```python
from build123d import *

# Parameters (mm, degrees)
ESTRUSIONE_ESTRUSIONE1_DEPTH    = 5
SCHIZZO5_R                      = 1.75
SCHIZZO5_R_2                    = 10
SCHIZZO5_R_3                    = 11
SCHIZZO5_R_4                    = 13
SCHIZZO5_R_5                    = 26
SCHIZZO5_W                      = 37
SCHIZZO5_H                      = 24
TAGLIO_ESTRUSIONE2_DEPTH        = 7
SCHIZZO6_R                      = 4
TAGLIO_ESTRUSIONE3_DEPTH        = 10
FORI_ALESATO_4_0MM1_D           = 4
FORI_ALESATO_4_0MM1_DEPTH       = 40.6
FORI_ALESATO_4_0MM1_CSINK_D     = 4.05
FORI_ALESATO_4_0MM1_CSINK_ANGLE = 90
FORI_ALESATO_4_0MM1_TIP         = 1.201721238


with BuildPart() as part:
    # Schizzo1 → Estrusione-Estrusione1 (new body)
    with BuildSketch(Plane.XY):
        with BuildLine():
            Line((0, 8), (0, 185))
            ThreePointArc((0, 185), (2.343145751, 190.656854249), (8, 193))
            Line((8, 193), (179, 193))
            ThreePointArc((179, 193), (184.656854249, 190.656854249), (187, 185))
            Line((187, 185), (187, 149.313708499))
            ThreePointArc((187, 149.313708499), (186.39103626, 146.25224104), (184.656854249, 143.656854249))
            Line((184.656854249, 143.656854249), (43.343145751, 2.343145751))
            ThreePointArc((43.343145751, 2.343145751), (40.74775896, 0.60896374), (37.686291501, 0))
            Line((37.686291501, 0), (8, 0))
            ThreePointArc((8, 0), (2.343145751, 2.343145751), (0, 8))
        make_face()
    extrude(amount=ESTRUSIONE_ESTRUSIONE1_DEPTH)

    # Schizzo5 → Taglio-Estrusione2 (cut)
    with BuildSketch(Plane.XY.offset(5)):
        with Locations((10, 90)):
            Circle(SCHIZZO5_R)
        with Locations((54.5, 90)):
            Circle(SCHIZZO5_R)
        with Locations((83.5, 161)):
            Circle(SCHIZZO5_R_2)
        with Locations((106.319509986, 90)):
            Circle(SCHIZZO5_R_3)
        with Locations((71.319509986, 90)):
            Circle(SCHIZZO5_R_4)
        with Locations((38, 138)):
            Circle(SCHIZZO5_R_5)
        with Locations((136, 138)):
            Circle(SCHIZZO5_R_5)
        with Locations((38, 42)):
            Circle(SCHIZZO5_R_5)
        with Locations((83.5, 127.850051573)):
            Circle(SCHIZZO5_R_2)
        with Locations((32.25, 90)):
            Rectangle(SCHIZZO5_W, SCHIZZO5_H)
    extrude(amount=-TAGLIO_ESTRUSIONE2_DEPTH, mode=Mode.SUBTRACT)

    # Schizzo6 → Taglio-Estrusione3 (cut)
    with BuildSketch(Plane.XY.offset(5)):
        with Locations((22, 173)):
            Circle(SCHIZZO6_R)
        with Locations((66, 173)):
            Circle(SCHIZZO6_R)
        with Locations((121, 173)):
            Circle(SCHIZZO6_R)
        with Locations((165, 173)):
            Circle(SCHIZZO6_R)
    extrude(amount=-TAGLIO_ESTRUSIONE3_DEPTH, mode=Mode.SUBTRACT)

    # Fori Alesato Ø4.0mm1
    with Locations(Plane(origin=(0, 0, 0), x_dir=(-1, 0, 0), z_dir=(0, 0, -1))):
        with Locations((-182.36, 149.12), (-7.5, 185.4), (-39.69, 3.83)):
            CounterSinkHole(FORI_ALESATO_4_0MM1_D / 2, FORI_ALESATO_4_0MM1_CSINK_D / 2, depth=FORI_ALESATO_4_0MM1_DEPTH, counter_sink_angle=FORI_ALESATO_4_0MM1_CSINK_ANGLE)
            with Locations((0, 0, -(FORI_ALESATO_4_0MM1_DEPTH + FORI_ALESATO_4_0MM1_TIP / 2))):  # 118° drill point
                Cone(0, FORI_ALESATO_4_0MM1_D / 2, FORI_ALESATO_4_0MM1_TIP, mode=Mode.SUBTRACT)


solid = part.part
```
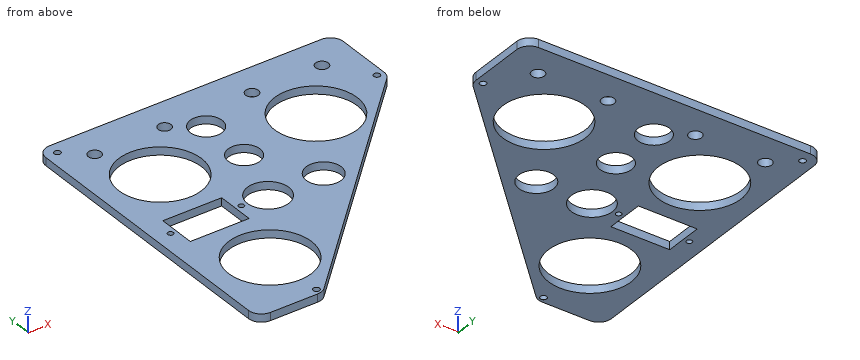
The model under review builds one solid part; all positions refer to its coordinate system, in mm. Give positions to 0.01 mm unless a question says otherwise; leave off trailing zeros. Write each loop counter-clockwise with the first axis right and the second up, starting at its lowest first coordinate (ties: lowest second). Pieces come first, ordered by that corner, then holes. Notation, with made-up numbers: (12.25, -6.75) -> (65.25, -6.75) arc R18 cw to (65.25, 23.25) -> close; hole circle Ø3 at (-32, -37). An arc over 180 degrees is marked (long way). Answer in a Markdown table with one row per item.
1) Add section B-B on y = 115.5. State the section outline as (x, z) points.
Worked answers:
| item | result |
|---|---|
| outline | (0, 0) -> (24.97, 0) -> (24.97, 5) -> (0, 5) -> close; (51.03, 0) -> (122.97, 0) -> (122.97, 5) -> (51.03, 5) -> close; (149.03, 0) -> (156.5, 0) -> (156.5, 5) -> (149.03, 5) -> close |
2) Add section A-A on x = 146. State the section outline as (y, z) points, plus the area to 3 significant figures.
Worked answers:
| item | result |
|---|---|
| outline | (105, 0) -> (114, 0) -> (114, 5) -> (105, 5) -> close; (162, 0) -> (193, 0) -> (193, 5) -> (162, 5) -> close |
| area | 200 mm² |
3) Clearance check with flat-ended pins moving along their axes: P1, Ø1, axis at y = 29.5, z = 4, coming from the +X side; P2, Ø5, axis at x = 66, y = 173, coming from the +Z side; P3, Ø1.5, axis at y = 87, z = 1.5, coming from the +X side. State where each tip first meets the part, or that it passes through.
Worked answers:
| item | result |
|---|---|
| P1 | x = 71 |
| P2 | through |
| P3 | x = 128.75 |
4) Add section D-D on y = 158. State the section outline as (x, z) points, plus the area to 3 significant figures.
Worked answers:
| item | result |
|---|---|
| outline | (0, 0) -> (21.39, 0) -> (21.39, 5) -> (0, 5) -> close; (54.61, 0) -> (73.96, 0) -> (73.96, 5) -> (54.61, 5) -> close; (93.04, 0) -> (119.39, 0) -> (119.39, 5) -> (93.04, 5) -> close; (152.61, 0) -> (187, 0) -> (187, 5) -> (152.61, 5) -> close |
| area | 507 mm² |
5) Add section C-C on x = 121. State the section outline as (y, z) points.
Worked answers:
| item | result |
|---|---|
| outline | (80, 0) -> (116.76, 0) -> (116.76, 5) -> (80, 5) -> close; (159.24, 0) -> (169, 0) -> (169, 5) -> (159.24, 5) -> close; (177, 0) -> (193, 0) -> (193, 5) -> (177, 5) -> close |
6) For L1, parallel to X at y = 132, z = 4.75; L2, parallel to Y at x = 49, z = 4.7; L3, parallel to Y at x = 42.5, z = 3.65, list the stretches that pass through material, from the lowest coordinate up. Write a range as [from, to].
Worked answers:
| item | result |
|---|---|
| L1 | [0, 12.7], [63.3, 74.4], [92.6, 110.7], [161.3, 173] |
| L2 | [8, 18.44], [65.56, 78], [102, 114.44], [161.56, 193] |
| L3 | [1.61, 16.39], [67.61, 78], [102, 112.39], [163.61, 193] |
